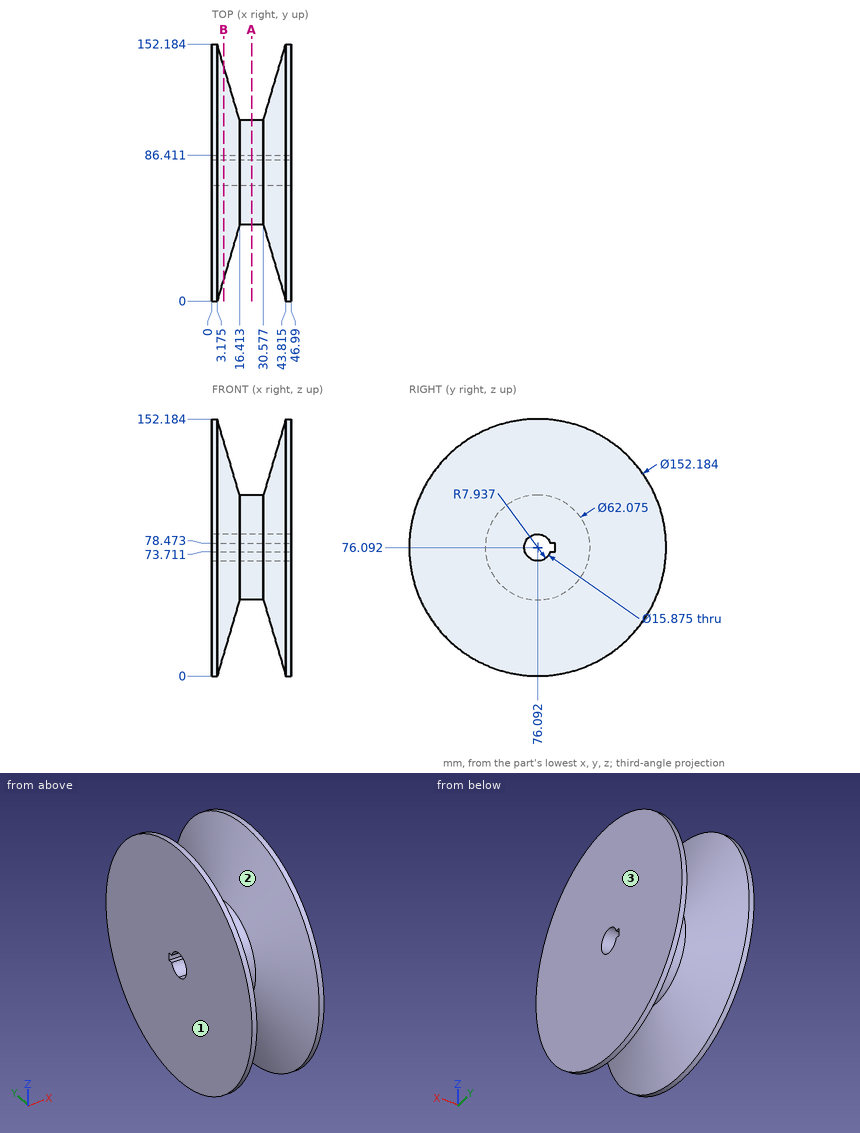
Drawing for the job (mm, zero at the part's lowest x, y, z). Round coordinates to 2 decimals unless told otherwise and drop trailing zeros. Loops run counter-clockwise (first coordinate to the right, second up) from the corner with the lowest first, then second, coordinate; pieces in that order, holes last. Notation, with made-up numbers: M -14,-4 L -3,-4 A13 cw -3,3 Z; hole C 11.25,59 d1. An arc over 180 degrees is marked long. Use a Markdown table: item, result. Add a question column.
(1) Drill centre lines: line 1 (X direction, y = 137, z = 121); line 2 (X direction, y = 90, z = 138.5) (1 decimal); line 3 (Y direction, x = 18, z = 100) (1 decimal). Where is each one in solid material? Low to high.
(2) Pull direction X, two halves, no side cores. Call the marked faces 1, 2 and 3: +X half, -X half, draft (parallel to the pull), parting line (faces both ways), or undercut.
(3) Flat gauge pins, fed straight in: pin 1 (5 mm diameter, centred on x = 5, z = 42.5, fed in from +Y); pin 2 (2 mm diameter, centred on x = 25.5, y = 85, fed in from +Z) (1 decimal). Where does each tip first touch, or does it go through?
(4) Cut at A-A (x = 23.5). Give the cut face in (y, z) (1 decimal), and give its area (3 significant figures).
(5) Cut at B-B (x = 7). Give the cut face in (y, z) (1 decimal), and give its area (3 significant figures).
Geometry says:
| question | item | result |
|---|---|---|
| 1 | line 1 | x = 0 to 3.3, 43.69 to 46.99 |
| 1 | line 2 | x = 0 to 6.7, 40.2 to 47 |
| 1 | line 3 | y = 56.3 to 95.9 |
| 2 | face 1 | -X half |
| 2 | face 2 | undercut |
| 2 | face 3 | +X half |
| 3 | pin 1 | stops at y = 145.18 |
| 3 | pin 2 | stops at z = 106.1 |
| 4 | outline | C 76.1,76.1 d62.1; hole M 83.7,73.7 L 86.4,73.7 L 86.4,78.5 L 83.7,78.5 A7.9 ccw long Z |
| 4 | area | 2,820 mm² |
| 5 | outline | C 76.1,76.1 d126.1; hole M 83.7,73.7 L 86.4,73.7 L 86.4,78.5 L 83.7,78.5 A7.9 ccw long Z |
| 5 | area | 12,300 mm² |
